Read the model definition and answer for the solid it produces. Units are mm, in the model's axes. Face numbers are marked on the shaded views. A direction names the side the tool comes from. Coordinates: 2 decimals unless noted, no trailing zeros. Order: outer loops, then holes, each group sorted by start corner. A loop starts at its lowest first (then second) coordinate and runs counter-clockwise, first axis right, second up. Notation, with made-up numbers: (62.25, 12) -> (106.25, 12) arc R11 ccw to (106.25, 17) -> close; hole circle Ø9 at (37.25, -23). An arc over 180 degrees is marked (long way). Answer as a JSON object with one key per item and string values. Group by question number.
1) Consider L1, parallel to Z at x = 2.25, y = 0.1; L2, parallel to X at y = -2, z = -0.3; L3, parallel to Z at x = 6, y = 0.1. Determine where each line is inside the solid, lowest interval first.
2) Determine the mould class of the marked faces 4, 5 and 6 for opening direction Y: released by +Y, released by -Y, zero draft, split by the parting line, or undercut.
3) Section A-A on x = 4 is taken. Determine the outline of the cut face in (y, z).
4) Given pin 1 (2 mm diameter, centred on x = 8, y = 1, fed in from +Z); pin 2 (1.5 mm diameter, centred on x = 2.5, z = 1.5, fed in from -Y); pin 3 (2 mm diameter, centred on x = 6.5, z = -2, fed in from -Y), each flat-ended and moving along its own axis, determine where each tip first touches the part or whether it passes through.
5) A tool of negligible diameter and unlimited length cuts with its end or side. For the marked faces 1, 2 and 3, from which of +Z, -Z, +X, -X, +Y, -Y can it reach the whole face along a straight path? Write none if from no direction.
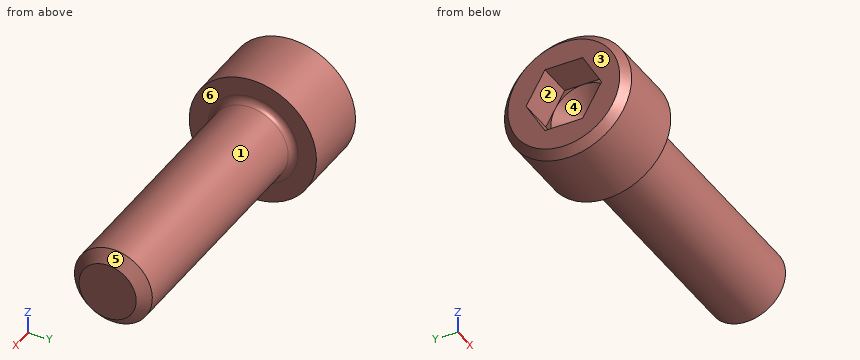
from build123d import *

# Parameters (mm, degrees)
FILLET1_R   = 0.2286
HEX_2_DEPTH = 1.2954


with BuildPart() as part:
    # BodySke → Base-Revolve (revolve)
    with BuildSketch(Plane.XY, mode=Mode.PRIVATE) as base_revolve_sk:
        Polygon((0, 0), (0, 2.0447), (0.2794, 2.3241), (2.8448, 2.3241), (2.8448, 1.4224), (11.99134, 1.4224), (12.3698, 1.04394), (12.3698, 0), align=None)
    revolve(base_revolve_sk.sketch.rotate(Axis((-31.75, 0, 0), (1, 0, 0)), 90), axis=Axis((-31.75, 0, 0), (1, 0, 0)))

    # Fillet1
    fillet1_edges = [part.edges().sort_by_distance(p)[0] for p in [
        (2.8448, 0, -1.4224),
    ]]
    fillet(fillet1_edges, radius=FILLET1_R)

    # Sketch2 → Hex-PreBroach (revolve, cut)
    with BuildSketch(Plane.XY, mode=Mode.PRIVATE) as hex_prebroach_sk:
        Polygon((0, 1.1938), (1.2954, 1.1938), (1.984640751, 0), (0, 0), align=None)
    revolve(hex_prebroach_sk.sketch.rotate(Axis((0, 0, 0), (1, 0, 0)), 90), axis=Axis((0, 0, 0), (1, 0, 0)), mode=Mode.SUBTRACT)

    # Sketch3 → Hex 2 (cut)
    with BuildSketch(Plane(origin=(0, 0, 0), x_dir=(0, 0.500000000000001, 0.866025403784438), z_dir=(-1, 0, 0))):
        Polygon((0.689240751, 1.1938), (-0.689240751, 1.1938), (-1.378481503, 0), (-0.689240751, -1.1938), (0.689240751, -1.1938), (1.378481503, 0), align=None)
    extrude(amount=-HEX_2_DEPTH, mode=Mode.SUBTRACT)


solid = part.part
Worked answers:
{
 "1": {"L1": "z = -2.32 to 2.32", "L2": "x = 0 to 2.84", "L3": "z = -1.42 to 1.42"},
 "2": {"face 4": "undercut", "face 5": "split by the parting line", "face 6": "zero draft"},
 "3": {"outline": "circle Ø2.84 at (0, 0)"},
 "4": {"pin 1": "stops at z = 1.42", "pin 2": "stops at y = -2.2", "pin 3": "stops at y = -1.01"},
 "5": {"face 1": "+X", "face 2": "-X", "face 3": "+Z, -Z, -X, +Y, -Y"}
}
